```python
from build123d import *

# Parameters (mm, degrees)
SKETCH1_R           = 14
BOSS_EXTRUDE1_DEPTH = 4
SKETCH2_R           = 14
SKETCH2_R_2         = 6.5
CUT_EXTRUDE1_DEPTH  = 0.5
SKETCH3_R           = 1.65
CUT_EXTRUDE2_DEPTH  = 4


with BuildPart() as part:
    # Sketch1 → Boss-Extrude1 (new body)
    with BuildSketch(Plane(origin=(0, 0, 0), x_dir=(1, 0, 0), z_dir=(0, 1, 0))):
        Circle(SKETCH1_R)
    extrude(amount=BOSS_EXTRUDE1_DEPTH)

    # Sketch2 → Cut-Extrude1 (cut)
    with BuildSketch(Plane.XZ):
        Circle(SKETCH2_R)
        Circle(SKETCH2_R_2, mode=Mode.SUBTRACT)
    extrude(amount=-CUT_EXTRUDE1_DEPTH, mode=Mode.SUBTRACT)

    # Sketch3 → Cut-Extrude2 (cut)
    with BuildSketch(Plane(origin=(0, 4, 0), x_dir=(1, 0, 0), z_dir=(0, 1, 0))):
        Circle(SKETCH3_R)
    extrude(amount=-CUT_EXTRUDE2_DEPTH, mode=Mode.SUBTRACT)


solid = part.part
```
Source: CAD feature listing. Evaluate the final solid. Frame: model axes, mm. Round coordinates to 2 decimals unless told otherwise and drop trailing zeros. Loops run counter-clockwise (first coordinate to the right, second up) from the corner with the lowest first, then second, coordinate; pieces in that order, holes last. Notation, with made-up numbers: M -6,15 L 36,15 A28 cw 36,51 Z; hole C 0,86.25 d11. An arc over 180 degrees is marked long. Put each result on its own line as item: value.
(1) Section D-D, the plane z = -5.25. Return loops of the section in (x, y).
Solutions:
outline: M -12.98,0.5 L -3.83,0.5 L -3.83,0 L 3.83,0 L 3.83,0.5 L 12.98,0.5 L 12.98,4 L -12.98,4 Z
(2) Pull-direction query (X, two-part tool) for faces 1 (the face through (3, 0.5, -6)), 2 (the face through (-1.216, 2.028, -1.115)), 3 (the face through (-5.158, 0.246, -3.955)); classes: released by +X, released by -X, zero draft, split by the parting line, or undercut.
Solutions:
face 1: zero draft
face 2: undercut
face 3: split by the parting line
(3) Ray query, line 1 (X direction, y = 0.8, z = 0); line 2 (Y direction, x = 6.25, z = 12). Return the intervals inside material, ascending. Write a range as [from, to].
Solutions:
line 1: [-14, -1.65], [1.65, 14]
line 2: [0.5, 4]
(4) Section A-A, the plane z = 0. Return loops of the section in (x, y), and give its area (3 significant figures).
Solutions:
outline: M -14,0.5 L -6.5,0.5 L -6.5,0 L -1.65,0 L -1.65,4 L -14,4 Z; M 1.65,0 L 6.5,0 L 6.5,0.5 L 14,0.5 L 14,4 L 1.65,4 Z
area: 91.3 mm²
(5) Section B-B, the plane x = 0. Return loops of the section in (y, z), and give its area (3 significant figures).
Solutions:
outline: M 0,-6.5 L 0.5,-6.5 L 0.5,-14 L 4,-14 L 4,-1.65 L 0,-1.65 Z; M 0,1.65 L 4,1.65 L 4,14 L 0.5,14 L 0.5,6.5 L 0,6.5 Z
area: 91.3 mm²
(6) First-contact query: pin 1 (2.5 mm diameter, centred on x = 0, z = 0, fed in from -Y). Flat tip, straight axial feed; report the tip coordinate or a pass-through.
Solutions:
pin 1: through
(7) Section C-C, the plane y = 2.5. Return loops of the section in (x, z).
Solutions:
outline: C 0,0 d28; hole C 0,0 d3.3
